Here's how the part is built. I have some questions about the finished solid (model axes, mm). Face numbers are marked on the shaded views. A direction names the side the tool comes from. Round coordinates to 2 decimals unless told otherwise and drop trailing zeros. Write each loop counter-clockwise with the first axis right and the second up, starting at its lowest first coordinate (ties: lowest second). Pieces come first, ordered by that corner, then holes. Notation, with made-up numbers: M 39,76.5 L 55,76.5 A32 cw 55,102.5 Z; hole C 54,81 d11. An arc over 180 degrees is marked long. Write item = value, one per line. Start each with the question number.
(1) I want a section at B-B (x = -28.5). List the corners of the cut face in (y, z) for me, and give its area (3 significant figures).
(2) On a 3-axis mill with a long thin cutter (end or side, diameter ignored), from which of +Z, -Z, +X, -X, +Y, -Y can I reach the whole of each face in a straight line? I mean the marked faces 1 and 2. Say none if no direction works.
(3) I want a section at D-D (y = -40.5). List the corners of the cut face in (x, z) for me.
(4) I need wall thicknesses on line 1 along X through (y, z) = (11, 80); line 2 along Z through (x, y) = (56, 29.5); line 3 along Y through (x, z) = (17, 67.5). Which ranges of each line are inside material? Lowest first, please.
(5) I want a section at A-A (y = 2). List the corners of the cut face in (x, z) for me.
(6) Will these pins go through, and if not, where does the flat tip stop? pin 1 Ø2 at (x, z) = (38, 48.5) entering from -Y; pin 2 Ø12 at (x, y) = (38, 35.5) entering from +Z; pin 3 Ø19.5 at (y, z) = (32.5, 84) entering from +X.
(7) I want a section at C-C (z = 30.5). List the corners of the cut face in (x, y) for me.
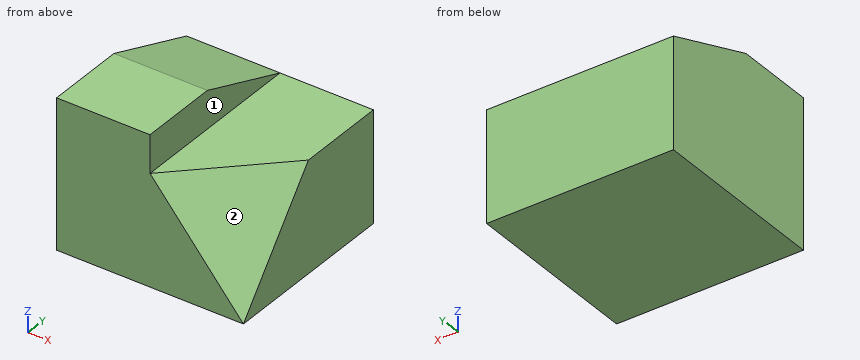
```python
from build123d import *

# Parameters (mm, degrees)
F0_W     = 121.8784451485
F0_H     = 118.6291240156
F1_DEPTH = 72.39
F3_DEPTH = 60.96
F7_DEPTH = 49.1183372137


with BuildPart() as f1:
    # F0 (on Top) → F1 (new body)
    with BuildSketch(Plane.XY):
        with Locations((1.138780266, 7.0254523307)):
            Rectangle(F0_W, F0_H)
    extrude(amount=F1_DEPTH)

    # F2 (on face) → F3 (join)
    with BuildSketch(Plane(origin=(-59.8004423082, 0, 0), x_dir=(0, -1, 0), z_dir=(-1, 0, 0))):
        Polygon((-66.3400143385, 72.39), (52.2891096771, 72.39), (52.2891096771, 97.0183685422), (0, 97.0183685422), align=None)
    extrude(amount=-F3_DEPTH)

    # F6 (on 3pt) → F7 (cut, through all)
    with BuildSketch(Plane(origin=(41.9043027589, -43.0374073868, 35.2637791007), x_dir=(-0.7987945895, -0.4653434391, 0.3812908174), z_dir=(-0.6016038595, 0.6178714042, -0.5062684309))):
        Polygon((-25.255178673, 60.4466734116), (-25.255178673, -33.1403415326), (51.0077879865, 22.8536668575), align=None)
    extrude(amount=-F7_DEPTH, mode=Mode.SUBTRACT)


solid = f1.part
```
Returned:
q1.outline = M -52.29,0 L 66.34,0 L 66.34,72.39 L 0,97.02 L -52.29,97.02 Z
q1.area = 10,700 mm²
q2.face_1 = +Z, +X, +Y, -Y
q2.face_2 = +Z, +X, -Y
q3.outline = M -59.8,0 L 62.08,0 L 62.08,14.39 L 13.27,72.39 L 1.16,72.39 L 1.16,97.02 L -59.8,97.02 Z
q4.line_1 = -59.8 to 1.16
q4.line_2 = 0 to 72.39
q4.line_3 = -40.87 to 66.34
q5.outline = M -59.8,0 L 62.08,0 L 62.08,66.26 L 56.92,72.39 L 1.16,72.39 L 1.16,96.28 L -59.8,96.28 Z
q6.pin_1 = -37.27
q6.pin_2 = 72.39
q6.pin_3 = 1.16
q7.outline = M -59.8,-52.29 L 36.41,-52.29 L 62.08,-27.3 L 62.08,66.34 L -59.8,66.34 Z
